from build123d import *

# Parameters (mm, degrees)
SKETCH_1_W          = 104
SKETCH_1_H          = 96
EXTRUDE_1_DEPTH     = 2
SKETCH_2_W          = 2
SKETCH_2_H          = 96
EXTRUDE_2_DEPTH     = 26
SKETCH_3_R          = 1.75
CUT_EXTRUDE_1_DEPTH = 116.689238912
SKETCH_4_W          = 26
SKETCH_4_H          = 56.5
CUT_EXTRUDE_2_DEPTH = 118.45637488
FILLET_2_R          = 1
SKETCH_5_W          = 6
SKETCH_5_H          = 14.25
CUT_EXTRUDE_3_DEPTH = 118.45637488
SKETCH_6_W          = 4.5
SKETCH_6_H          = 1
EXTRUDE_3_DEPTH     = 12.65
SKETCH_7_R          = 1.25
CUT_EXTRUDE_4_DEPTH = 111.526015037


with BuildPart() as part:
    # 草图1 → 凸台-拉伸1 (new body)
    with BuildSketch(Plane.XY):
        Rectangle(SKETCH_1_W, SKETCH_1_H)
    extrude(amount=EXTRUDE_1_DEPTH)

    # 草图2 → 凸台-拉伸2 (add)
    with BuildSketch(Plane(origin=(0, 0, 0), x_dir=(-1, 0, 0), z_dir=(0, 0, -1))):
        with Locations((-51, 0)):
            Rectangle(SKETCH_2_W, SKETCH_2_H)
    extrude(amount=EXTRUDE_2_DEPTH)

    # 草图3 → 切除-拉伸1 (cut, through all)
    with BuildSketch(Plane.ZY.offset(-50)):
        with Locations((-5, 44.5)):
            Circle(SKETCH_3_R)
        with Locations((-5, 38)):
            Circle(SKETCH_3_R)
        with Locations((-5, 31.5)):
            Circle(SKETCH_3_R)
        with Locations(Location((-21, 31.5, 0), (0, 0, 180))):
            Circle(SKETCH_3_R)
        with Locations(Location((-21, 38, 0), (0, 0, 180))):
            Circle(SKETCH_3_R)
        with Locations(Location((-21, 44.5, 0), (0, 0, 180))):
            Circle(SKETCH_3_R)
        with Locations((-21, -44.5)):
            Circle(SKETCH_3_R)
        with Locations((-21, -38)):
            Circle(SKETCH_3_R)
        with Locations((-21, -31.5)):
            Circle(SKETCH_3_R)
        with Locations(Location((-5, -31.5, 0), (0, 0, 180))):
            Circle(SKETCH_3_R)
        with Locations(Location((-5, -38, 0), (0, 0, 180))):
            Circle(SKETCH_3_R)
        with Locations(Location((-5, -44.5, 0), (0, 0, 180))):
            Circle(SKETCH_3_R)
    extrude(amount=-CUT_EXTRUDE_1_DEPTH, mode=Mode.SUBTRACT)

    # 草图4 → 切除-拉伸2 (cut, through all)
    with BuildSketch(Plane(origin=(52, 0, 0), x_dir=(0, 0, -1), z_dir=(1, 0, 0))):
        with Locations((13, 0)):
            Rectangle(SKETCH_4_W, SKETCH_4_H)
    extrude(amount=-CUT_EXTRUDE_2_DEPTH, mode=Mode.SUBTRACT)

    # 圆角2
    fillet_2_edges = [part.edges().sort_by_distance(p)[0] for p in [
        (50, -38.125, 0),
        (50, 38.125, 0),
    ]]
    fillet(fillet_2_edges, radius=FILLET_2_R)

    # 草图5 → 切除-拉伸3 (cut, through all)
    with BuildSketch(Plane(origin=(52, 0, 0), x_dir=(0, 0, -1), z_dir=(1, 0, 0))):
        with Locations((13, 35.375)):
            Rectangle(SKETCH_5_W, SKETCH_5_H)
        with BuildLine():
            ThreePointArc((10, 42.5), (13, 45.5), (16, 42.5))
            Line((16, 42.5), (10, 42.5))
        make_face()
        with Locations((13, -35.375)):
            Rectangle(SKETCH_5_W, SKETCH_5_H)
        with BuildLine():
            Line((10, -42.5), (16, -42.5))
            ThreePointArc((16, -42.5), (13, -45.5), (10, -42.5))
        make_face()
    extrude(amount=-CUT_EXTRUDE_3_DEPTH, mode=Mode.SUBTRACT)

    # 草图6 → 凸台-拉伸3 (add)
    with BuildSketch(Plane(origin=(0, 0, 0), x_dir=(-1, 0, 0), z_dir=(0, 0, -1))):
        with Locations((49.75, 45.5)):
            Rectangle(SKETCH_6_W, SKETCH_6_H)
    extrude_3 = extrude(amount=EXTRUDE_3_DEPTH)

    # 草图7 → 切除-拉伸4 (cut, through all)
    with BuildSketch(Plane(origin=(0, 46, 0), x_dir=(1, 0, 0), z_dir=(0, 1, 0))):
        with Locations(Location((-49.75, 6.325, 0), (0, 0, 180))):
            Circle(SKETCH_7_R)
    cut_extrude_4 = extrude(amount=-CUT_EXTRUDE_4_DEPTH, mode=Mode.SUBTRACT)

    # 镜向1: 凸台-拉伸3, 切除-拉伸4 across plane
    add(extrude_3.mirror(Plane.ZX))
    add(cut_extrude_4.mirror(Plane.ZX), mode=Mode.SUBTRACT)


solid = part.part
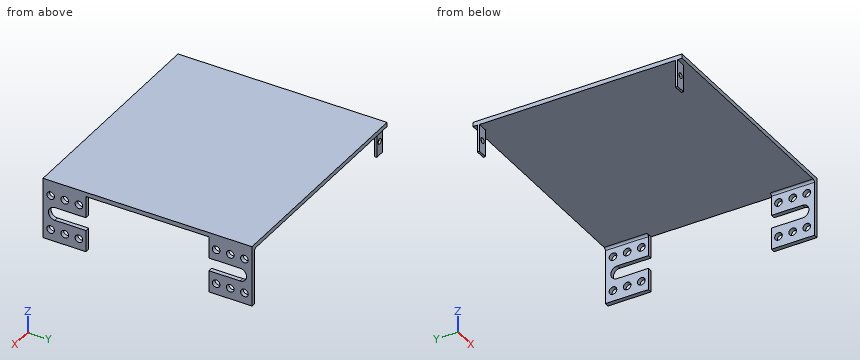
Read the model definition and answer for the solid it produces. Units are mm, in the model's axes. Round coordinates to 2 decimals unless told otherwise and drop trailing zeros. Order: outer loops, then holes, each group sorted by start corner. A loop starts at its lowest first (then second) coordinate and runs counter-clockwise, first axis right, second up.
1) Flat-ended cylindrical pins translate along their axes: pin 1 (4.5 mm diameter, centred on y = 38, z = -21, fed in from +X); pin 2 (1.3 mm diameter, centred on x = -49.5, z = -9, fed in from +Y); pin 3 (3 mm diameter, centred on y = -44.5, z = -5, fed in from +X); pin 4 (12 mm diameter, centred on x = 34, y = 31, fed in from -Z). Find the tip coordinate at first contact, or state that the pin passes through.
2) The part is cut by section C-C on z = -21. Give the number of separate pieces and of enclosed holes in the cut face, plus the area to 3 significant figures.
3) The part is cut by section B-B on x = -49.75. Write down the section's boundary in (y, z) (3 decimals).
4) The part is cut by section A-A on y = -38. Write down the section's boundary in (x, z), plus the area to 3 significant figures.
5) Straight lines are drawn through the part: L1, parallel to Z at x = 47.5, y = -15; L2, parallel to X at y = 35.5, z = -5.75. For each, find the intervals that lie inside material, in ascending order.
6) The part is cut by section D-D on x = 3.5. Write down the section's boundary in (y, z).
Resolved:
1. pin 1: stops at x = 52
1. pin 2: stops at y = 46
1. pin 3: stops at x = -47.5
1. pin 4: stops at z = 0
2. separate pieces: 8
2. enclosed holes: 0
2. area: 37.0 mm2
3. outline: (-48, 0) - (-46, 0) - (-46, -5.075) - (-45, -5.075) - (-45, 0) - (45, 0) - (45, -5.075) - (46, -5.075) - (46, 0) - (48, 0) - (48, 2) - (-48, 2) - close; (-46, -12.65) - (-45, -12.65) - (-45, -7.575) - (-46, -7.575) - close; (45, -12.65) - (46, -12.65) - (46, -7.575) - (45, -7.575) - close
4. outline: (-52, 0) - (49, 0) arc R1 cw to (50, -1) - (50, -3.25) - (52, -3.25) - (52, 2) - (-52, 2) - close; (50, -26) - (52, -26) - (52, -22.75) - (50, -22.75) - close; (50, -19.25) - (52, -19.25) - (52, -16) - (50, -16) - close; (50, -10) - (52, -10) - (52, -6.75) - (50, -6.75) - close
4. area: 234 mm2
5. L1: z = 0 to 2
5. L2: x = 50 to 52
6. outline: (-48, 0) - (48, 0) - (48, 2) - (-48, 2) - close
